For this review, take the finished solid that the model builds, in its own axes (mm). A direction names the side the tool comes from. Round coordinates to 2 decimals unless told otherwise and drop trailing zeros. Order: outer loops, then holes, each group sorted by start corner. A loop starts at its lowest first (then second) coordinate and runs counter-clockwise, first axis right, second up. Notation, with made-up numbers: (-10, -39) -> (47, -39) arc R11 cw to (47, -34) -> close; hole circle Ø1 at (68, 81). An arc over 180 degrees is marked (long way). Use a Markdown table: item, result. Add a question column.
1) Consider section A-A (z = 22). State the section outline as (x, y) points, plus the area to 3 significant figures.
2) Machinability: for faces 1 (the face through (18, 0, 47.968)), 2 (the face through (10.428, 0, 15)), 3 (the face through (7.773, 0, 16)), 4 (the face through (13, -7.584, 35)), 5 (the face through (9, 0, 0)), which of the approach directions +Z, -Z, +X, -X, +Y, -Y give a long, thin tool a straight path to every point of the face, cutting with its end or side? Answer none if there is none.
3) Draft analysis for pull direction Y (two halves, no side actions). For faces 6 (the face through (17, 0, 50.622)), 7 (the face through (11, 10.807, 31)), 8 (the face through (12, 7.584, 35)), state which applies: pulls with the +Y half, pulls with the -Y half, needs draft (parallel to the pull), parting line crosses it, or undercut.
4) Consider section B-B (y = 0.5). State the section outline as (x, z) points.
5) Wall thickness on line 1 along X through (y, z) = (0.75, 19); line 2 along Y through (x, z) = (1, 18); line 3 along Z through (x, y) = (39, -3.75): over which ranges is each line inside the solid? List them lowest first. Write a range as [from, to].
6) Consider section C-C (x = 36.5). State the section outline as (y, z) points.
7) Consider section D-D (x = 1.5). State the section outline as (y, z) points.
8) Clearance check with a flat-ended pin moving along its axis: P1, Ø4, axis at y = -7.5, z = 12, coming from the +X side. State where the tip first meets the part, or that it passes through.
```python
from build123d import *

# Parameters (mm, degrees)
F1_W   = 20.855685696
F1_H   = 21.614074707
F1_W_2 = 15.5469644815
F1_H_2 = 15.1677737013


with BuildPart() as f2:
    # F2: sweep along a path in F0
    with BuildLine(Plane.XZ) as f2_path:
        Line((0, 0), (0, 40.1945970953))
        Line((0, 40.1945970953), (43.6073467135, 40.1945970953))
    # F1 (on Top) → F2 (sweep)
    with BuildSketch(Plane.XY):
        Rectangle(F1_W, F1_H)
        Rectangle(F1_W_2, F1_H_2, mode=Mode.SUBTRACT)
    sweep(path=f2_path.line, transition=Transition.RIGHT)


solid = f2.part
```
Results list:
| question | item | result |
|---|---|---|
| 1 | outline | (-10.43, -10.81) -> (10.43, -10.81) -> (10.43, 10.81) -> (-10.43, 10.81) -> close; hole (-7.77, -7.58) -> (7.77, -7.58) -> (7.77, 7.58) -> (-7.77, 7.58) -> close |
| 1 | area | 215 mm2 |
| 2 | face 1 | +X |
| 2 | face 2 | -Z, +X, +Y, -Y |
| 2 | face 3 | -Z |
| 2 | face 4 | none |
| 2 | face 5 | -Z, +X, -X, +Y, -Y |
| 3 | face 6 | needs draft |
| 3 | face 7 | pulls with the +Y half |
| 3 | face 8 | undercut |
| 4 | outline | (-10.43, 0) -> (-7.77, 0) -> (-7.77, 47.97) -> (43.61, 47.97) -> (43.61, 50.62) -> (-10.43, 50.62) -> close; (7.77, 0) -> (10.43, 0) -> (10.43, 29.77) -> (43.61, 29.77) -> (43.61, 32.42) -> (7.77, 32.42) -> close |
| 5 | line 1 | [-10.43, -7.77], [7.77, 10.43] |
| 5 | line 2 | [-10.81, -7.58], [7.58, 10.81] |
| 5 | line 3 | [29.77, 32.42], [47.97, 50.62] |
| 6 | outline | (-10.81, 29.77) -> (10.81, 29.77) -> (10.81, 50.62) -> (-10.81, 50.62) -> close; hole (-7.58, 32.42) -> (7.58, 32.42) -> (7.58, 47.97) -> (-7.58, 47.97) -> close |
| 7 | outline | (-10.81, 0) -> (-7.58, 0) -> (-7.58, 47.97) -> (7.58, 47.97) -> (7.58, 0) -> (10.81, 0) -> (10.81, 50.62) -> (-10.81, 50.62) -> close |
| 8 | P1 | x = 10.43 |
